Source: CAD feature listing. Evaluate the final solid. Frame: model axes, mm. Face numbers are marked on the shaded views. A direction names the side the tool comes from. Give positions to 0.01 mm unless a question says otherwise; leave off trailing zeros. Loops run counter-clockwise (first coordinate to the right, second up) from the corner with the lowest first, then second, coordinate; pieces in that order, holes last. Notation, with made-up numbers: M 79.5,-5.75 L 122.5,-5.75 A17 ccw 122.5,6.25 Z; hole C -4,74.25 d4. An arc over 180 degrees is marked long. Put each result on its own line as item: value. Start each with the question number.
Autodesk Inventor part; units mm, degrees
ref_plane "YZ Plane" through (0, 0, 0) normal (1, 0, 0) x (0, 1, 0)
ref_plane "XZ Plane" through (0, 0, 0) normal (0, 1, 0) x (-1, 0, 0)
ref_plane "XY Plane" through (0, 0, 0) normal (0, 0, 1) x (1, 0, 0)
sketch "Sketch1" plane through (0, 0, 0) normal (0, 1, 0) x (-1, 0, 0)
  line L0 (50, 100) -> (-50, 100)
  line L1 (-50, 100) -> (-50, -100)
  line L2 (-50, -100) -> (50, -100)
  line L3 (50, -100) -> (50, 100)
  line L4 (50, 100) -> (-50, -100) construction
  line L5 (-50, 100) -> (50, -100) construction
  line L6 (-47, -97) -> (47, -97)
  line L7 (47, -97) -> (47, 97)
  line L8 (47, 97) -> (-47, 97)
  line L9 (-47, 97) -> (-47, -97)
  line L10 (-47, -97) -> (47, 97) construction
  line L11 (47, -97) -> (-47, 97) construction
  line L12 (50, 100) -> (50, 77)
  line L13 (50, 77) -> (-50, 77)
  line L14 (0, 0) -> (10.1877, 0)
  line L15 (50, -77) -> (-50, -77)
  line L16 (0, 0) -> (0, -5.3943)
  line L17 (0, 100) -> (0, -100)
  line L18 (47, 97) -> (31.3333, 97)
  circle A0 centre (39.1667, 86.2777) radius 5
  line L19 (39.1667, 86.2777) -> (47, 86.2777)
  line L20 (39.1667, 86.2777) -> (31.3333, 86.2777)
  line L21 (31.3333, 86.2777) -> (31.3333, 77)
  line L22 (31.3333, 97) -> (31.3333, 86.2777)
  line L23 (0, 0) -> (-10.1877, 0)
  circle A1 centre (-39.1667, 86.2777) radius 5
  line L24 (-31.3333, 86.2777) -> (-31.3333, 77)
  line L25 (-31.3333, 97) -> (-31.3333, 86.2777)
  circle A2 centre (39.1667, -86.2777) radius 5
  line L26 (31.3333, -86.2777) -> (31.3333, -77)
  line L27 (31.3333, -97) -> (31.3333, -86.2777)
  circle A3 centre (-39.1667, -86.2777) radius 5
  line L28 (-31.3333, -86.2777) -> (-31.3333, -77)
  line L29 (-31.3333, -97) -> (-31.3333, -86.2777)
  line L30 (-31.3333, 77) -> (-31.3333, -77)
  line L31 (31.3333, 77) -> (31.3333, -77)
  line L32 (39.1667, 86.2777) -> (39.1667, -86.2777)
  line L33 (-39.1667, 86.2777) -> (-39.1667, -86.2777)
  line L34 (50, 77) -> (50, 74)
  line L35 (50, 74) -> (31.3333, 74)
  line L36 (50, -77) -> (50, -74)
  line L37 (50, -74) -> (31.3333, -74)
  line L38 (-31.3333, 77) -> (-31.3333, 74)
  line L39 (-31.3333, 74) -> (-50, 74)
  line L40 (-50, -77) -> (-50, -74)
  line L41 (-50, -74) -> (-31.3333, -74)
  dimension "d0" = 100
  dimension "d1" = 200
  dimension "d2" = 94
  dimension "d3" = 194
  dimension "d4" = 23
  dimension "d6" = 10
  dimension "d7" = 7.8333
  dimension "d8" = 7.8333
  dimension "d11" = 3
  dimension "d12" = 3
  dimension "d13" = 3
  dimension "d14" = 3
extrude "Extrusion1" add sketch "Sketch1" along normal blind 3 contours L3 L13 L7 L8 L17 L0 | L17 L8 L9 L13 L1 L0 | L3 L35 L7 L13 | L17 L13 L24 L25 L8 | L8 L22 L21 L13 L17 | L13 L32 A0 L19 L7 | L7 L35 L32 L13 | L13 L9 L39 L1 | L8 L7 L19 A0 L20 L22 | L25 L24 L13 L9 L8 | L17 L16 L15 L30 L13 | L13 L31 L15 L17 L16 | L3 L15 L7 L37 | L32 L35 L31 L13 | L13 L21 L20 A0 L32 | L13 L33 L39 L9 | L30 L39 L33 L13 | L3 L2 L17 L6 L7 L15 | L7 L15 L32 L37 | L41 L9 L15 L1 | L7 L6 L27 L26 L15 | L32 L15 L31 L37 | L15 L9 L6 L17 L2 L1 | L41 L33 L15 L9 | L30 L15 L33 L41 | L17 L6 L29 L28 L15 | L15 L26 L27 L6 L17 | L15 L28 L29 L6 L9
sketch "Sketch2" plane through (0, 0, 0) normal (0, -1, 0) x (1, 0, 0)
  line L0 (50, -74) -> (50, -100)
  line L1 (31.3333, -74) -> (50, -74)
  line L2 (31.3333, 74) -> (31.3333, -74)
  line L3 (50, 74) -> (31.3333, 74)
  line L4 (50, 100) -> (50, 74)
  line L5 (-50, 100) -> (50, 100)
  line L6 (-50, 74) -> (-50, 100)
  line L7 (-31.3333, 74) -> (-50, 74)
  line L8 (-31.3333, -74) -> (-31.3333, 74)
  line L9 (-50, -74) -> (-31.3333, -74)
  line L10 (-50, -100) -> (-50, -74)
  line L11 (50, -100) -> (-50, -100)
  line L12 (28.3333, -77) -> (47, -77)
  line L13 (47, -77) -> (47, -97)
  line L14 (47, -97) -> (-47, -97)
  line L15 (-47, -97) -> (-47, -77)
  line L16 (-47, -77) -> (-28.3333, -77)
  line L17 (-28.3333, -77) -> (-28.3333, 77)
  line L18 (-28.3333, 77) -> (-47, 77)
  line L19 (-47, 77) -> (-47, 97)
  line L20 (-47, 97) -> (47, 97)
  line L21 (47, 97) -> (47, 77)
  line L22 (47, 77) -> (28.3333, 77)
  line L23 (28.3333, 77) -> (28.3333, -77)
  point P0 (0, 0)
  dimension "d15" = 3
extrude "Extrusion2" add sketch "Sketch2" along normal blind 30
sketch "Sketch3" plane through (0, -30, 0) normal (0, -1, 0) x (1, 0, 0)
  line L0 (31.3333, 74) -> (50, 74)
  line L1 (50, 74) -> (50, 100)
  line L2 (50, 100) -> (-50, 100)
  line L3 (-50, 100) -> (-50, 74)
  line L4 (-50, 74) -> (-31.3333, 74)
  line L5 (-31.3333, -74) -> (-50, -74)
  line L6 (-50, -74) -> (-50, -100)
  line L7 (-50, -100) -> (50, -100)
  line L8 (50, -100) -> (50, -74)
  line L9 (50, -74) -> (31.3333, -74)
  line L10 (28.3333, -77) -> (47, -77)
  line L11 (47, -77) -> (47, -97)
  line L12 (47, -97) -> (-47, -97)
  line L13 (-47, -97) -> (-47, -77)
  line L14 (-47, -77) -> (-28.3333, -77)
  line L15 (-28.3333, -77) -> (-28.3333, 77)
  line L16 (-28.3333, 77) -> (-47, 77)
  line L17 (-47, 77) -> (-47, 97)
  line L18 (-47, 97) -> (47, 97)
  line L19 (47, 97) -> (47, 77)
  line L20 (47, 77) -> (28.3333, 77)
  line L21 (28.3333, 77) -> (28.3333, -77)
  line L22 (31.3333, 74) -> (-50, 74)
  line L23 (31.3333, -74) -> (-50, -74)
  point P0 (0, 0)
  point P1 (28.3333, -74)
  point P2 (-28.3333, -74)
  point P3 (-28.3333, 74)
  point P4 (28.3333, 74)
extrude "Extrusion3" add sketch "Sketch3" along normal blind 20 contours L22 L21 L20 L19 L18 L17 L16 L15 L4 L3 L2 L1 L0 | L23 L9 L8 L7 L6 L5 L15 L14 L13 L12 L11 L10 L21
sketch "Sketch4" plane through (0, 0, 0) normal (0, -1, 0) x (1, 0, 0)
  line L0 (28.3333, 77) -> (47, 77)
  line L1 (47, 77) -> (47, 97)
  line L2 (47, 97) -> (-47, 97)
  line L3 (-47, 97) -> (-47, 77)
  line L4 (-47, 77) -> (-28.3333, 77)
  line L5 (-28.3333, -77) -> (-47, -77)
  line L6 (-47, -77) -> (-47, -97)
  line L7 (-47, -97) -> (47, -97)
  line L8 (47, -97) -> (47, -77)
  line L9 (47, -77) -> (28.3333, -77)
  circle A0 centre (39.1667, -86.2777) radius 5
  circle A1 centre (39.1667, 86.2777) radius 5
  circle A2 centre (-39.1667, -86.2777) radius 5
  circle A3 centre (-39.1667, 86.2777) radius 5
  line L10 (28.3333, 77) -> (28.3333, 97)
  line L11 (-28.3333, 77) -> (-28.3333, 97)
  line L12 (-28.3333, -77) -> (-28.3333, -97)
  line L13 (28.3333, -77) -> (28.3333, -97)
  point P0 (0, 0)
extrude "Extrusion4" add sketch "Sketch4" along normal up to surface (50 mm away)
properties part number "atas"
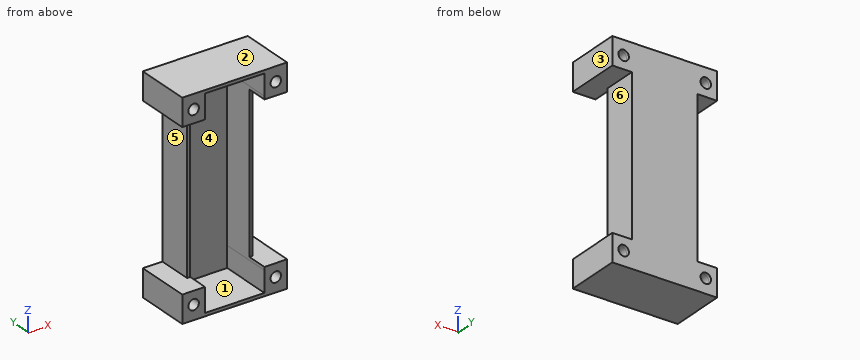
1. Ray query, line 1 (Z direction, x = -39, y = -17); line 2 (Z direction, x = 46.5, y = -15.5); line 3 (X direction, y = -8, z = 46.5). Return the intervals inside material, ascending.
2. Set-up query: the marked faces 4, 5 and 6. Return all of +Z, -Z, +X, -X, +Y, -Y with unobstructed straight access to the full face (end or side cutting, diameter ignored); none if empty.
3. Section C-C, the plane x = 18.5. Output: boundary loops of the cut face in (y, z), plus the area to 3 significant figures.
4. Section D-D, the plane y = -8. Output: boundary loops of the cut face in (x, z).
5. Section A-A, the plane y = -37. Output: boundary loops of the cut face in (x, z).
6. Section B-B, the plane z = -3.5. Output: boundary loops of the cut face in (x, y).
7. Pull-direction query (Z, two-part tool) for the marked faces 1, 2 and 3; classes: released by +Z, released by -Z, zero draft, split by the parting line, or undercut.
8. Contact query for flat-ended pins moving along their axis: pin 1 (25 mm diameter, centred on y = -21, z = -31.5, fed in from -X); pin 2 (1.5 mm diameter, centred on x = -30, z = 1.5, fed in from -Y); pin 3 (6 mm diameter, centred on x = 39.17, z = -86.28, fed in from +Y); pin 4 (1 mm diameter, centred on y = -11, z = 11, fed in from +X). Output: stop coordinate, or through.
Results found:
1. line 1: -100 to -91.27, -81.28 to -74, 74 to 81.28, 91.27 to 100
1. line 2: -100 to -74, 74 to 100
1. line 3: -31.33 to -28.33, 28.33 to 31.33
2. face 4: -Y
2. face 5: -X, +Y, -Y
2. face 6: +X, +Y, -Y
3. outline: M -50,-100 L 3,-100 L 3,100 L -50,100 L -50,97 L 0,97 L 0,-97 L -50,-97 Z
3. area: 900 mm²
4. outline: M -50,-100 L 50,-100 L 50,-74 L 31.33,-74 L 31.33,74 L 50,74 L 50,100 L -50,100 L -50,74 L -31.33,74 L -31.33,-74 L -50,-74 Z; hole C -39.17,-86.28 d10; hole C -39.17,86.28 d10; hole M -28.33,-97 L 28.33,-97 L 28.33,97 L -28.33,97 Z; hole C 39.17,-86.28 d10; hole C 39.17,86.28 d10
5. outline: M -50,-100 L 50,-100 L 50,-74 L 28.33,-74 L 28.33,-97 L -28.33,-97 L -28.33,-74 L -50,-74 Z; M -50,74 L -28.33,74 L -28.33,97 L 28.33,97 L 28.33,74 L 50,74 L 50,100 L -50,100 Z; hole C -39.17,-86.28 d10; hole C -39.17,86.28 d10; hole C 39.17,-86.28 d10; hole C 39.17,86.28 d10
6. outline: M -31.33,-30 L -28.33,-30 L -28.33,0 L 28.33,0 L 28.33,-30 L 31.33,-30 L 31.33,3 L -31.33,3 Z
7. face 1: undercut
7. face 2: released by +Z
7. face 3: zero draft
8. pin 1: x = -31.33
8. pin 2: y = -30
8. pin 3: through
8. pin 4: x = 31.33
